Source: CAD feature listing. Evaluate the final solid. Frame: model axes, mm. A direction names the side the tool comes from. Coordinates: 2 decimals unless noted, no trailing zeros. Write each loop counter-clockwise with the first axis right and the second up, starting at its lowest first coordinate (ties: lowest second). Pieces come first, ordered by that corner, then holes. Notation, with made-up numbers: (-21, 50.25) - (-13, 50.25) arc R12 ccw to (-13, 60.25) - close; hole circle Ø8 at (-25, 21). An arc over 180 degrees is marked (long way). One line per item, written item: value.
from build123d import *

# Parameters (mm, degrees)
SKETCH1_W               = 152.4
SKETCH1_H               = 76.2
BOSS_EXTRUDE1_DEPTH     = 50.8
SKETCH1_3_W             = 152.4
SKETCH1_3_H             = 76.2
BOSS_EXTRUDE2_DEPTH     = 3.175
SKETCH8_W               = 152.4
SKETCH8_H               = 47.625
CUT_EXTRUDE1_DEPTH      = 6.35
BOSS_EXTRUDE10_REACH    = 212.462
BOSS_EXTRUDE11_DEPTH    = 3.175
SKETCH12_W              = 34.925
SKETCH12_H              = 38.1
BOSS_EXTRUDE12_DEPTH    = 3.175
CUT_EXTRUDE2_DEPTH      = 153.300748931
CUT_EXTRUDE2_DEPTH_BACK = 153.300748931
SKETCH13_W              = 34.925
SKETCH13_H              = 12.7
SKETCH14_W              = 34.925
SKETCH14_H              = 85.725
CUT_EXTRUDE3_DEPTH      = 12.7
CUT_EXTRUDE4_DEPTH      = 6.096
CUT_EXTRUDE4_DEPTH_BACK = 173.99
SKETCH16_R              = 3.81
SKETCH17_W              = 165.1
SKETCH17_H              = 82.55
CUT_EXTRUDE5_DEPTH      = 3.175
SKETCH25_W              = 6.35
SKETCH25_H              = 6.35
BOSS_EXTRUDE16_DEPTH    = 44.45
FILLET2_R               = 8.89
FILLET3_R               = 1.27
CUT_EXTRUDE8_DEPTH      = 150.562384559
CUT_EXTRUDE8_DEPTH_BACK = 150.562384559
SKETCH26_R              = 1.27
FILLET4_R               = 3.048
CUT_EXTRUDE9_DEPTH      = 176.173701579
CUT_EXTRUDE9_DEPTH_BACK = 7.366
SKETCH27_R              = 6.35
FILLET5_R               = 3.048


with BuildPart() as part:
    # Sketch1 → Boss-Extrude1 (new body)
    with BuildSketch(Plane(origin=(0, 0, 0), x_dir=(1, 0, 0), z_dir=(0, 1, 0))):
        Polygon((-117.475, 41.275), (-117.475, -41.275), (-114.3, -41.275), (-114.3, 38.1), (-82.55, 38.1), (-82.55, -41.275), (82.55, -41.275), (82.55, 38.1), (114.3, 38.1), (114.3, -41.275), (117.475, -41.275), (117.475, 41.275), align=None)
        Rectangle(SKETCH1_W, SKETCH1_H, mode=Mode.SUBTRACT)
    extrude(amount=BOSS_EXTRUDE1_DEPTH)

    # Sketch1<3> → Boss-Extrude2 (add)
    with BuildSketch(Plane(origin=(0, 0, 0), x_dir=(1, 0, 0), z_dir=(0, 1, 0))):
        Rectangle(SKETCH1_3_W, SKETCH1_3_H)
    extrude(amount=BOSS_EXTRUDE2_DEPTH)

    # Sketch8 → Cut-Extrude1 (cut)
    with BuildSketch(Plane.XY.offset(41.275)):
        with Locations((0, 26.9875)):
            Rectangle(SKETCH8_W, SKETCH8_H)
    extrude(amount=-CUT_EXTRUDE1_DEPTH, mode=Mode.SUBTRACT)

    # Boss-Extrude10: up to this face of the body (flat: up to its plane)
    boss_extrude10_end = Plane(part.part.faces().sort_by_distance((82.55, 25.4, 1.5875))[0])
    # Sketch10 → Boss-Extrude10 (add, up to the picked face)
    with BuildSketch(Plane.ZY.offset(82.55), mode=Mode.PRIVATE) as boss_extrude10_sk1:
        Polygon((41.275, 50.8), (79.375, 0), (41.275, 0), (41.275, 3.175), (73.025, 3.175), (41.275, 45.508333333), align=None)
    boss_extrude10_tool1 = split(extrude(boss_extrude10_sk1.sketch, amount=-BOSS_EXTRUDE10_REACH, mode=Mode.PRIVATE), bisect_by=boss_extrude10_end, keep=Keep.BOTH, mode=Mode.PRIVATE)
    add(boss_extrude10_tool1.solids().sort_by(Axis((-82.55, 25.019, 59.817), (1, 0, 0)))[0])

    # Sketch11 → Boss-Extrude11 (add)
    with BuildSketch(Plane(origin=(82.55, 0, 0), x_dir=(0, 0, -1), z_dir=(1, 0, 0))):
        Polygon((-41.275, 45.508333333), (-73.025, 3.175), (-41.275, 3.175), align=None)
    boss_extrude11 = extrude(amount=-BOSS_EXTRUDE11_DEPTH)

    # Sketch12 → Boss-Extrude12 (add)
    with BuildSketch(Plane.XY.offset(41.275)):
        with Locations((100.0125, 19.05)):
            Rectangle(SKETCH12_W, SKETCH12_H)
    boss_extrude12 = extrude(amount=BOSS_EXTRUDE12_DEPTH)

    # Mirror2: Boss-Extrude11 across plane
    add(boss_extrude11.mirror(Plane(origin=(0, 0, 0), x_dir=(0, 0, 1), z_dir=(1, 0, 0))))

    # Mirror3: Boss-Extrude12 across plane
    add(boss_extrude12.mirror(Plane(origin=(0, 0, 0), x_dir=(0, 0, 1), z_dir=(1, 0, 0))))

    # Sketch13 → Cut-Extrude2 (cut, two sides: drawn at the far end of the back side and taken through both)
    with BuildSketch(Plane.XY.offset(41.275).offset(-CUT_EXTRUDE2_DEPTH_BACK)):
        with Locations((100.0125, 44.45)):
            Rectangle(SKETCH13_W, SKETCH13_H)
        with Locations((-100.0125, 44.45)):
            Rectangle(SKETCH13_W, SKETCH13_H)
    extrude(amount=CUT_EXTRUDE2_DEPTH + CUT_EXTRUDE2_DEPTH_BACK, mode=Mode.SUBTRACT)

    # Sketch14 → Cut-Extrude3 (cut)
    with BuildSketch(Plane(origin=(0, 0, 0), x_dir=(-1, 0, 0), z_dir=(0, -1, 0))):
        with Locations((-100.0125, -1.5875)):
            Rectangle(SKETCH14_W, SKETCH14_H)
    cut_extrude3 = extrude(amount=-CUT_EXTRUDE3_DEPTH, mode=Mode.SUBTRACT)

    # Mirror4: Cut-Extrude3 across plane
    add(cut_extrude3.mirror(Plane(origin=(0, 0, 0), x_dir=(0, 0, 1), z_dir=(1, 0, 0))), mode=Mode.SUBTRACT)

    # Sketch16 → Cut-Extrude4 (cut, two sides: drawn at the far end of the back side and taken through both)
    with BuildSketch(Plane.ZY.offset(82.55).offset(-CUT_EXTRUDE4_DEPTH_BACK)):
        with Locations(Location((-3.175, 20.066, 0), (0, 0, 180))):
            Circle(SKETCH16_R)
    extrude(amount=CUT_EXTRUDE4_DEPTH + CUT_EXTRUDE4_DEPTH_BACK, mode=Mode.SUBTRACT)

    # Sketch17 → Cut-Extrude5 (cut)
    with BuildSketch(Plane(origin=(0, 50.8, 0), x_dir=(1, 0, 0), z_dir=(0, 1, 0))):
        Rectangle(SKETCH17_W, SKETCH17_H)
    extrude(amount=-CUT_EXTRUDE5_DEPTH, mode=Mode.SUBTRACT)

    # Sketch25 → Boss-Extrude16 (add)
    with BuildSketch(Plane(origin=(0, 3.175, 0), x_dir=(1, 0, 0), z_dir=(0, 1, 0))):
        with Locations((73.025, -38.1)):
            Rectangle(SKETCH25_W, SKETCH25_H)
        with Locations((-73.025, -38.1)):
            Rectangle(SKETCH25_W, SKETCH25_H)
    extrude(amount=BOSS_EXTRUDE16_DEPTH)

    # Fillet2
    # the kernel refuses this fillet: 8.89 mm, written as the material it adds along each edge
    with BuildSketch(Plane(origin=(76.2, 3.175, 34.925), x_dir=(0, 0, -1), z_dir=(0, 1, 0))) as fillet2_piece_1:
        with BuildLine():
            CenterArc((8.519418994, 8.89), FILLET2_R, 196.601549599, 73.398450401)
            Line((0, 6.35), (-0.17038838, 6.2992))
            ThreePointArc((-0.17038838, 6.2992), (-0.1778, 3.175), (-0.1778, 0))
            Line((-0.1778, 0), (0, -0.1778))
            Line((0, -0.1778), (8.519418994, -0.1778))
            Line((8.519418994, -0.1778), (8.519418994, 0))
        make_face()
    extrude(amount=44.45)
    with BuildSketch(Plane(origin=(76.2, 3.175, -38.1), x_dir=(-1, 0, 0), z_dir=(0, 1, 0)), Plane(origin=(-76.2, 3.175, -38.1), x_dir=(0, 0, 1), z_dir=(0, 1, 0))) as fillet2_piece_2:
        with BuildLine():
            CenterArc((FILLET2_R, FILLET2_R), FILLET2_R, 180, 90)
            Line((0, FILLET2_R), (-FILLET2_R * 0.02, FILLET2_R))
            Line((-FILLET2_R * 0.02, FILLET2_R), (-FILLET2_R * 0.02, -FILLET2_R * 0.02))
            Line((-FILLET2_R * 0.02, -FILLET2_R * 0.02), (FILLET2_R, -FILLET2_R * 0.02))
            Line((FILLET2_R, -FILLET2_R * 0.02), (FILLET2_R, 0))
        make_face()
    extrude(amount=44.45)
    with BuildSketch(Plane(origin=(-76.2, 3.175, 34.925), x_dir=(1, 0, 0), z_dir=(0, 1, 0))) as fillet2_piece_3:
        with BuildLine():
            CenterArc((8.89, 8.519418994), FILLET2_R, 180, 73.398450401)
            Line((0, 8.519418994), (-0.1778, 8.519418994))
            Line((-0.1778, 8.519418994), (-0.1778, 0))
            Line((-0.1778, 0), (0, -0.1778))
            ThreePointArc((0, -0.1778), (3.175, -0.1778), (6.2992, -0.17038838))
            Line((6.2992, -0.17038838), (6.35, 0))
        make_face()
    extrude(amount=44.45)

    # Fillet3
    fillet3_edges = [part.edges().sort_by_distance(p)[0] for p in [
        (74.6125, 3.175, 41.275),
        (79.375, 3.175, 57.15),
        (0, 3.175, 73.025),
        (-79.375, 3.175, 57.15),
        (-74.6125, 3.175, 41.275),
        (-69.85, 3.175, 38.1),
        (-74.437857322, 3.175, 31.718372174),
        (-76.2, 3.175, -1.402209497),
        (-73.596179285, 3.175, -35.496179285),
        (0, 3.175, -38.1),
        (73.596179285, 3.175, -35.496179285),
        (76.2, 3.175, -1.402209497),
        (74.437857322, 3.175, 31.718372174),
        (69.85, 3.175, 38.1),
        (-69.85, 25.4, 34.925),
        (69.85, 25.4, 34.925),
        (0, 50.8, 41.275),
    ]]
    fillet(fillet3_edges, radius=FILLET3_R)

    # Sketch26 → Cut-Extrude8 (cut, two sides: drawn at the far end of the back side and taken through both)
    with BuildSketch(Plane(origin=(0, 47.625, 0), x_dir=(1, 0, 0), z_dir=(0, 1, 0)).offset(-CUT_EXTRUDE8_DEPTH_BACK)):
        with Locations(Location((-76.2, 34.925, 0), (0, 0, 270))):
            Circle(SKETCH26_R)
        with Locations(Location((76.2, 34.925, 0), (0, 0, 270))):
            Circle(SKETCH26_R)
        with Locations(Location((76.271823643, -34.767866531, 0), (0, 0, 270))):
            Circle(SKETCH26_R)
        with Locations(Location((-76.127852634, -35.081985097, 0), (0, 0, 270))):
            Circle(SKETCH26_R)
    extrude(amount=CUT_EXTRUDE8_DEPTH + CUT_EXTRUDE8_DEPTH_BACK, mode=Mode.SUBTRACT)

    # Fillet4
    fillet4_edges = [part.edges().sort_by_distance(p)[0] for p in [
        (-114.3, 25.4, 41.275),
        (-114.3, 25.4, -38.1),
        (-82.55, 25.4, -38.1),
        (-82.55, 25.4, 41.275),
        (82.55, 25.4, 41.275),
        (114.3, 25.4, 41.275),
        (114.3, 25.4, -38.1),
        (82.55, 25.4, -38.1),
        (82.55, 12.7, 42.8625),
        (-82.55, 12.7, 42.8625),
        (-82.55, 38.1, 42.8625),
        (82.55, 38.1, 42.8625),
        (117.475, 25.4, -41.275),
        (117.475, 25.4, 44.45),
        (82.55, 25.4, 44.45),
        (-117.475, 25.4, 44.45),
        (-82.55, 25.4, 44.45),
        (-117.475, 25.4, -41.275),
        (-82.55, 6.35, -41.275),
        (82.55, 6.35, -41.275),
        (82.55, 42.8625, -41.275),
        (-82.55, 42.8625, -41.275),
    ]]
    fillet(fillet4_edges, radius=FILLET4_R)

    # Sketch27 → Cut-Extrude9 (cut, two sides: drawn at the far end of the back side and taken through both)
    with BuildSketch(Plane(origin=(0, 0, -41.275), x_dir=(-1, 0, 0), z_dir=(0, 0, -1)).offset(-CUT_EXTRUDE9_DEPTH_BACK)):
        with Locations((0, 46.99)):
            Circle(SKETCH27_R)
    extrude(amount=CUT_EXTRUDE9_DEPTH + CUT_EXTRUDE9_DEPTH_BACK, mode=Mode.SUBTRACT)

    # Fillet5
    fillet5_edges = [part.edges().sort_by_distance(p)[0] for p in [
        (6.318170226, 47.625, -39.6875),
        (-6.318170226, 47.625, -39.6875),
    ]]
    fillet(fillet5_edges, radius=FILLET5_R)


solid = part.part
1) Contact query for flat-ended pins moving along their axis: P1, Ø12, axis at x = 43, z = 24.5, coming from the +Y side (3 decimals); P2, Ø19, axis at x = -102.5, z = 11.5, coming from the -Y side; P3, Ø4, axis at x = -16, y = 41.5, coming from the +Z side; P4, Ø7.5, axis at x = 76.5, y = 21.5, coming from the +Z side. Output: stop coordinate, or through.
Values found:
P1: y = 3.175
P2: through
P3: z = 49.75
P4: z = 66.06
2) Material intervals for line 1 (X direction, y = 30.5, z = 24.5) (3 decimals); line 2 (X direction, y = 34, z = 31) (3 decimals); line 3 (X direction, y = 20, z = 47.5) (3 decimals), sorted ascending.
Values found:
line 1: -117.475 to -114.3, -82.55 to -76.2, 76.2 to 82.55, 114.3 to 117.475
line 2: -117.475 to -114.3, -82.55 to -74.921, 74.921 to 82.55, 114.3 to 117.475
line 3: -82.55 to -79.375, 79.375 to 82.55
3) Reachability of faces 4 (the flat face through (-99, 25, -38.1)), 5 (the cylindrical face through (-79.33, 16.29, -2.68)), 6 (the cylindrical face through (0.12, 40.64, -39.67)), 7 (the flat face through (69.85, 26, 39)) from +Z, -Z, +X, -X, +Y, -Y: full face, straight path, thin tool, end or side. Return the list, or none.
Values found:
face 4: +Y, -Y
face 5: none
face 6: -Z, +Y
face 7: +Y
4) Section query A-A on z = -26. Output: boundary loops of the cut face in (x, y) (3 decimals).
Values found:
outline: (-117.475, 12.7) - (-114.3, 12.7) - (-114.3, 38.1) - (-117.475, 38.1) - close; (-82.55, 0) - (82.55, 0) - (82.55, 47.625) - (76.2, 47.625) - (76.2, 4.445) arc R1.27 cw to (74.93, 3.175) - (-74.93, 3.175) arc R1.27 cw to (-76.2, 4.445) - (-76.2, 47.625) - (-82.55, 47.625) - close; (114.3, 12.7) - (117.475, 12.7) - (117.475, 38.1) - (114.3, 38.1) - close
5) Section query B-B on x = 101.5. Output: boundary loops of the cut face in (y, z) (3 decimals), then the cut area to 3 significant figures.
Values found:
outline: (12.7, -41.275) - (38.1, -41.275) - (38.1, -38.1) - (12.7, -38.1) - close; (12.7, 41.275) - (38.1, 41.275) - (38.1, 44.45) - (12.7, 44.45) - close
area: 161 mm2
6) Draft query along Z for faces 1 (the flat face through (-114.3, 25, 2)), 2 (the flat face through (100, 26, 44.45)), 3 (the flat face through (-115, 12.7, 1)). Return one class per face: released by +Z, released by -Z, zero draft, split by the parting line, or undercut.
Values found:
face 1: undercut
face 2: released by +Z
face 3: zero draft
7) Section query C-C on x = 39. Output: boundary loops of the cut face in (y, z) (3 decimals), then the cut area to 3 significant figures.
Values found:
outline: (0, -41.275) - (47.625, -41.275) - (47.625, -38.1) - (4.445, -38.1) arc R1.27 cw to (3.175, -36.83) - (3.175, 70.485) arc R1.27 cw to (5.207, 71.501) - (45.508, 41.275) - (46.99, 41.275) arc R1.27 ccw to (47.752, 43.561) - (0, 79.375) - close
area: 698 mm2
